Source: CAD feature listing. Evaluate the final solid. Frame: model axes, mm. A direction names the side the tool comes from. Give positions to 0.01 mm unless a question says otherwise; leave off trailing zeros. Order: outer loops, then holes, each group sorted by start corner. A loop starts at its lowest first (then second) coordinate and runs counter-clockwise, first axis right, second up. Notation, with made-up numbers: M 21.25,27 L 25.25,27 A27 ccw 25.25,50 Z; hole C -23.75,54.25 d9. An arc over 180 degrees is marked long. Answer as a JSON object with one key per item and string values. Group by question number.
1. Section query D-D (z = 57). Output: boundary loops of the cut face in (x, y).
2. Section query C-C (x = 6). Output: boundary loops of the cut face in (y, z), plus the area to 3 significant figures.
3. Set-up query: faces 1 (the flat face through (-100, 75, 38.1)), 2 (the flat face through (102, 75, 38.1)), 3 (the flat face through (152.4, 75, 13)), 4 (the cylindrical face through (0.97, 75.13, 88.89)), 5 (the flat face through (-102, 38, 12.7)). Return all of +Z, -Z, +X, -X, +Y, -Y with unobstructed straight access to the full face (end or side cutting, diameter ignored); none if empty.
4. Material intervals for L1, parallel to Y at x = 101, z = 30; L2, parallel to X at y = 49.5, z = 35.5; L3, parallel to Y at x = 109, z = 28, sorted ascending. Write a range as [from, to].
5. Section query A-A (y = 63.5). Output: boundary loops of the cut face in (x, z), plus the area to 3 significant figures.
6. Pull-direction query (Y, two-part tool) for faces 6 (the flat face through (-2, 75, 0)), 7 (the flat face through (-2, 152.4, 6)), 8 (the cylindrical face through (107.46, 103.033, 25.578)); classes: +Y half, -Y half, draft (parallel to the pull), parting line (faces both ways), or undercut.
7. Pin query (flat end, axial travel): P1, Ø15, axis at x = -101.6, y = 114.3, coming from the +Z side; P2, Ø3, axis at x = 69.5, y = 86.5, coming from the +Z side; P3, Ø4, axis at y = 137, z = 28, coming from the -X side. Return the tip coordinate at first contact, or that it passes through.
8. Section query B-B (z = 33). Output: boundary loops of the cut face in (x, y), plus the area to 3 significant figures.
from build123d import *

# Parameters (mm, degrees)
F0_R     = 25.4
F1_DEPTH = 152.4
F2_R     = 12.7
F3_DEPTH = 25.4


with BuildPart() as f1:
    # F0 (on Front) → F1 (new body)
    with BuildSketch(Plane.XZ):
        with BuildLine():
            Line((-152.4, 25.4), (-152.4, 0))
            Line((-152.4, 0), (152.4, 0))
            Line((152.4, 0), (152.4, 25.4))
            ThreePointArc((152.4, 25.4), (148.680256, 34.380256), (139.7, 38.1))
            Line((139.7, 38.1), (62.217039, 38.1))
            ThreePointArc((62.217039, 38.1), (54.184854, 40.962622), (49.773632, 48.26))
            ThreePointArc((49.773632, 48.26), (0, 88.9), (-49.773632, 48.26))
            ThreePointArc((-49.773632, 48.26), (-54.184854, 40.962622), (-62.217039, 38.1))
            Line((-62.217039, 38.1), (-139.7, 38.1))
            ThreePointArc((-139.7, 38.1), (-148.680256, 34.380256), (-152.4, 25.4))
        make_face()
        with Locations((0, 38.1)):
            Circle(F0_R, mode=Mode.SUBTRACT)
    extrude(amount=-F1_DEPTH)

    # F2 (on face) → F3 (cut)
    with BuildSketch(Plane.XY.offset(38.1)):
        with Locations((-101.6, 114.3)):
            Circle(F2_R)
        with Locations((-101.6, 38.1)):
            Circle(F2_R)
        with Locations((101.6, 114.3)):
            Circle(F2_R)
        with Locations((101.6, 38.1)):
            Circle(F2_R)
    extrude(amount=-F3_DEPTH, mode=Mode.SUBTRACT)


solid = f1.part
Answer sheet:
{
 "1": {"outline": "M -47.15,0 L -16.97,0 L -16.97,152.4 L -47.15,152.4 Z; M 16.97,0 L 47.15,0 L 47.15,152.4 L 16.97,152.4 Z"},
 "2": {"outline": "M 0,0 L 152.4,0 L 152.4,13.42 L 0,13.42 Z; M 0,62.78 L 152.4,62.78 L 152.4,88.54 L 0,88.54 Z", "area": "5,970 mm^2"},
 "3": {"face 1": "+Z, -X, +Y, -Y", "face 2": "+Z, +X, +Y, -Y", "face 3": "+Z, -Z, +X, +Y, -Y", "face 4": "+Z, +Y, -Y", "face 5": "+Z"},
 "4": {"L1": "[0, 25.41], [50.79, 101.61], [126.99, 152.4]", "L2": "[-147.4, -107.2], [-96, -25.27], [25.27, 96], [107.2, 147.4]", "L3": "[0, 27.78], [48.42, 103.98], [124.62, 152.4]"},
 "5": {"outline": "M -152.4,0 L 152.4,0 L 152.4,25.4 A12.7 ccw 139.7,38.1 L 62.22,38.1 A12.7 cw 49.77,48.26 A50.8 ccw -49.77,48.26 A12.7 cw -62.22,38.1 L -139.7,38.1 A12.7 ccw -152.4,25.4 Z; hole C 0,38.1 d50.8", "area": "13,600 mm^2"},
 "6": {"face 6": "draft", "face 7": "+Y half", "face 8": "undercut"},
 "7": {"P1": "z = 12.7", "P2": "z = 38.1", "P3": "x = -152.39"},
 "8": {"outline": "M -149.87,0 L -24.88,0 L -24.88,152.4 L -149.87,152.4 Z; M 24.88,0 L 149.87,0 L 149.87,152.4 L 24.88,152.4 Z; hole C -101.6,38.1 d25.4; hole C -101.6,114.3 d25.4; hole C 101.6,38.1 d25.4; hole C 101.6,114.3 d25.4", "area": "36,100 mm^2"}
}
